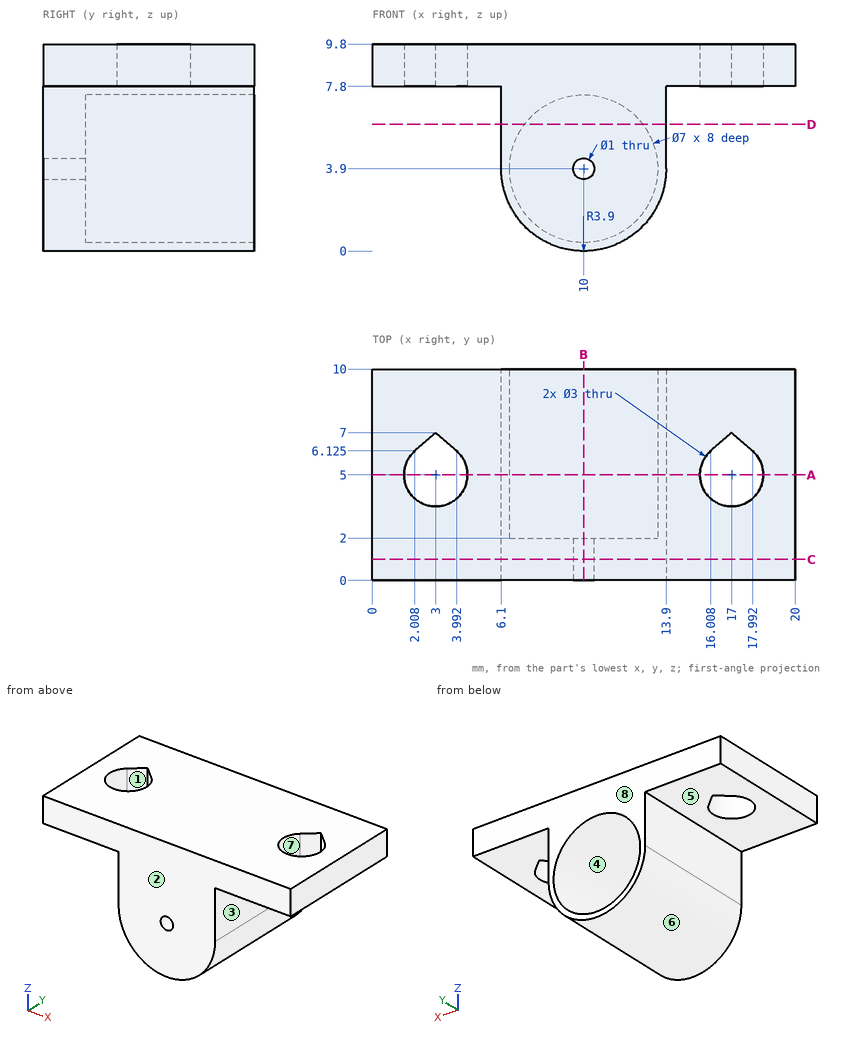
The figure shows three views and two pictorial views of one solid part (mm, origin at its lowest corner). Answer the questions. A direction names the side the tool comes from. Round coordinates to 2 decimals unless told otherwise and drop trailing zeros. Write each loop counter-clockwise with the first axis right and the second up, starting at its lowest first coordinate (ties: lowest second). Pieces come first, ordered by that corner, then holes. Notation, with made-up numbers: M 16.25,72.5 L 51.25,72.5 A20 ccw 51.25,78.5 Z; hole C 49.25,-29.5 d11. An arc over 180 degrees is marked long. Use a Markdown table: item, result.
1) The part is cut by section A-A on y = 5. Give the vertices of the cut face in (x, z).
Taken from the geometry:
| item | result |
|---|---|
| outline | M 0,7.8 L 1.5,7.8 L 1.5,9.8 L 0,9.8 Z; M 4.5,7.8 L 6.1,7.8 L 6.1,3.9 A3.9 ccw 13.9,3.9 L 13.9,7.8 L 15.5,7.8 L 15.5,9.8 L 4.5,9.8 Z; M 18.5,7.8 L 20,7.8 L 20,9.8 L 18.5,9.8 Z; hole C 10,3.9 d7 |
2) Which of the six approach directions +Z, -Z, +X, -X, +Y, -Y give full straight-line access (tool end or side, diameter ignored) to the marked faces 1, 2, 3, 4 and 5?
Taken from the geometry:
| item | result |
|---|---|
| face 1 | +Z, -Z |
| face 2 | +Z, -Z, +X, -X, -Y |
| face 3 | -Z, +X, +Y, -Y |
| face 4 | +Y |
| face 5 | -Z, -X, +Y, -Y |
3) The part is cut by section C-C on y = 1. Give the vertices of the cut face in (x, z).
Taken from the geometry:
| item | result |
|---|---|
| outline | M 0,7.8 L 6.1,7.8 L 6.1,3.9 A3.9 ccw 13.9,3.9 L 13.9,7.8 L 20,7.8 L 20,9.8 L 0,9.8 Z; hole C 10,3.9 d1 |
4) The part is cut by section D-D on z = 6. Give the vertices of the cut face in (x, y), plus the area to 3 significant figures.
Taken from the geometry:
| item | result |
|---|---|
| outline | M 6.1,0 L 13.9,0 L 13.9,10 L 12.8,10 L 12.8,2 L 7.2,2 L 7.2,10 L 6.1,10 Z |
| area | 33.2 mm2 |
5) The part is cut by section B-B on x = 10. Give the vertices of the cut face in (y, z).
Taken from the geometry:
| item | result |
|---|---|
| outline | M 0,0 L 10,0 L 10,0.4 L 2,0.4 L 2,3.4 L 0,3.4 Z; M 0,4.4 L 2,4.4 L 2,7.4 L 10,7.4 L 10,9.8 L 0,9.8 Z |
6) Flat-ended cylindrical pins translate along their axes: pin 1 (1.2 mm diameter, centred on y = 7, z = 6.5, fed in from +X); pin 2 (5 mm diameter, centred on x = 3, y = 5, fed in from -Z); pin 3 (5 mm diameter, centred on x = 4, y = 4.5, fed in from -Z). Find the tip coordinate at first contact, or state that the pin passes through.
Taken from the geometry:
| item | result |
|---|---|
| pin 1 | stops at x = 13.9 |
| pin 2 | stops at z = 7.8 |
| pin 3 | stops at z = 2.18 |
7) Consider line 1 (X direction, y = 5, z = 8.45); line 2 (X direction, y = 5.5, z = 8.75); line 3 (Z direction, x = 10, y = 0.7). Determine where each line is inside the solid, lowest interval first. Write a range as [from, to].
Taken from the geometry:
| item | result |
|---|---|
| line 1 | x = [0, 1.5], [4.5, 15.5], [18.5, 20] |
| line 2 | x = [0, 1.59], [4.41, 15.59], [18.41, 20] |
| line 3 | z = [0, 3.4], [4.4, 9.8] |
8) Determine the mould class of the marked faces 6, 7 and 8 for opening direction Y: pulls with the +Y half, pulls with the -Y half, needs draft (parallel to the pull), parting line crosses it, or undercut.
Taken from the geometry:
| item | result |
|---|---|
| face 6 | needs draft |
| face 7 | undercut |
| face 8 | pulls with the +Y half |
